Input: part model. Units: mm. Frame: model coordinates. A direction names the side the tool comes from. Round coordinates to 2 decimals unless told otherwise and drop trailing zeros. Order: outer loops, then holes, each group sorted by start corner. A loop starts at its lowest first (then second) coordinate and runs counter-clockwise, first axis right, second up. Notation, with made-up numbers: (-8.75, 84) -> (48.25, 84) arc R13 cw to (48.25, 90) -> close; hole circle Ø10 at (73.5, -5). An arc over 180 degrees is marked (long way). Use a Markdown table: item, result.
Autodesk Inventor part; units mm, degrees
ref_plane "YZ Plane" through (0, 0, 0) normal (1, 0, 0) x (0, 1, 0)
ref_plane "XZ Plane" through (0, 0, 0) normal (0, 1, 0) x (-1, 0, 0)
ref_plane "XY Plane" through (0, 0, 0) normal (0, 0, 1) x (1, 0, 0)
sketch "Эскиз1" plane through (0, 0, 0) normal (0, 0, 1) x (1, 0, 0)
  line L0 (0, 0) -> (-40, 0)
  line L1 (-40, -30) -> (-30, -30)
  line L2 (-30, -30) -> (-30, -34)
  line L3 (-30, -34) -> (-10, -34)
  line L4 (-10, -34) -> (-10, -30)
  line L5 (-10, -30) -> (0, -30)
  line L6 (-40, -30) -> (-40, -15)
  line L7 (-40, -15) -> (-32, -15)
  line L8 (-32, -15) -> (-32, 0)
  line L9 (-40, 30) -> (-30, 30)
  line L10 (-30, 30) -> (-30, 34)
  line L11 (-30, 34) -> (-10, 34)
  line L12 (-10, 34) -> (-10, 30)
  line L13 (-10, 30) -> (0, 30)
  line L14 (-40, 30) -> (-40, 15)
  line L15 (-40, 15) -> (-32, 15)
  line L16 (-32, 15) -> (-32, 0)
  line L17 (0, 30) -> (0, -30)
  line L18 (0, 0) -> (40, 0)
  line L19 (40, -30) -> (30, -30)
  line L20 (30, -30) -> (30, -34)
  line L21 (30, -34) -> (10, -34)
  line L22 (10, -34) -> (10, -30)
  line L23 (10, -30) -> (0, -30)
  line L24 (40, -30) -> (40, -15)
  line L25 (40, -15) -> (32, -15)
  line L26 (32, -15) -> (32, 0)
  line L27 (40, 30) -> (30, 30)
  line L28 (30, 30) -> (30, 34)
  line L29 (30, 34) -> (10, 34)
  line L30 (10, 34) -> (10, 30)
  line L31 (10, 30) -> (0, 30)
  line L32 (40, 30) -> (40, 15)
  line L33 (40, 15) -> (32, 15)
  line L34 (32, 15) -> (32, 0)
  dimension "d0" = 4
  dimension "d1" = 60
  dimension "d3" = 20
  dimension "d6" = 15
  dimension "d8" = 15
  dimension "d9" = 10
  dimension "d11" = 20
  dimension "d14" = 8
extrude "Выдавливание1" add sketch "Эскиз1" along normal blind 4
sketch "Эскиз2" plane through (0, 0, 4) normal (0, 0, 1) x (1, 0, 0)
  line L0 (10, 30) -> (-10, 30)
  line L1 (0, 30) -> (0, -30)
  line L2 (-10, -30) -> (10, -30)
  line L3 (-32, 15) -> (-32, -15)
  line L4 (-32, 0) -> (32, 0)
  line L5 (32, -15) -> (32, 15)
  line L6 (-40, 15) -> (-32, 15)
  line L7 (-30, 30) -> (-40, 30)
  line L8 (-40, 30) -> (-40, 15)
  point P0 (0, 0)
  point P1 (-36, -21)
  point P2 (36, -21)
  point P3 (-36, 21)
  point P4 (36, 21)
  point P5 (-36, 15)
  point P6 (-40, 22.5)
  dimension "d23" = 9
hole "Отверстие1" at (-36, -21, 4) at (36, -21, 4) at (-36, 21, 4) at (36, 21, 4) direction (0, 0, -1) diameter 3 end through all
sketch "Эскиз3" plane through (0, 0, 4) normal (0, 0, 1) x (1, 0, 0)
  line L0 (0, 0) -> (0, 30)
  line L1 (10, 30) -> (-10, 30)
  point P0 (-12.8, 10)
  point P1 (12.8, 10)
  dimension "d31" = 25.6
  dimension "d32" = 10
hole "Отверстие2" at (-12.8, 10, 4) at (12.8, 10, 4) direction (0, 0, -1) diameter 16 end through all
sketch "Эскиз4" plane through (0, 0, 4) normal (0, 0, 1) x (1, 0, 0)
  circle A0 centre (-12.8, 10) radius 8
  line L0 (-10, -30) -> (10, -30)
  line L1 (0, -30) -> (0, 30)
  line L2 (10, 30) -> (-10, 30)
  point P0 (0, 0)
  point P1 (-27.5, 10)
  point P2 (27.5, 10)
  dimension "d40" = 55
hole "Отверстие3" at (-27.5, 10, 4) at (27.5, 10, 4) direction (0, 0, -1) diameter 3 end through all
sketch "Эскиз5" plane through (0, 0, 4) normal (0, 0, 1) x (1, 0, 0)
  line L0 (-26, -3) -> (-3, -3)
  line L1 (-3, -3) -> (-3, -8)
  line L2 (-3, -8) -> (-26, -8)
  line L3 (-26, -8) -> (-26, -3)
  line L4 (3, -3) -> (26, -3)
  line L5 (26, -3) -> (26, -8)
  line L6 (26, -8) -> (3, -8)
  line L7 (3, -8) -> (3, -3)
  line L8 (-10, -30) -> (10, -30)
  line L9 (0, -30) -> (0, 30)
  line L10 (10, 30) -> (-10, 30)
  line L11 (32, -15) -> (32, 15)
  point P0 (0, 0)
  point P1 (3, -5.5)
  point P2 (-3, -5.5)
  dimension "d42" = 23
  dimension "d43" = 22
  dimension "d44" = 5
  dimension "d45" = 6
extrude "Выдавливание2" cut sketch "Эскиз5" against normal through all
properties part number "top" material "Дерево (береза)"
1) Cut plane A-A on y = 21. Return loops of the section in (x, z).
Answer key:
| item | result |
|---|---|
| outline | (-40, 0) -> (-37.5, 0) -> (-37.5, 4) -> (-40, 4) -> close; (-34.5, 0) -> (34.5, 0) -> (34.5, 4) -> (-34.5, 4) -> close; (37.5, 0) -> (40, 0) -> (40, 4) -> (37.5, 4) -> close |
2) Contact query for flat-ended pins moving along their axis: P1, Ø2.5, axis at x = 36, y = 21, coming from the -Z side; P2, Ø2, axis at y = -5, z = 3, coming from the +X side; P3, Ø1.2, axis at y = -6, z = 1, coming from the -X side; P4, Ø2, axis at y = 33, z = 2, coming from the +X side. Output: stop coordinate, or through.
Answer key:
| item | result |
|---|---|
| P1 | passes through |
| P2 | stops at x = 32 |
| P3 | stops at x = -32 |
| P4 | stops at x = 30 |
3) Cut plane B-B on x = 36. Return loops of the section in (y, z), and give its area (3 significant figures).
Answer key:
| item | result |
|---|---|
| outline | (-30, 0) -> (-22.5, 0) -> (-22.5, 4) -> (-30, 4) -> close; (-19.5, 0) -> (-15, 0) -> (-15, 4) -> (-19.5, 4) -> close; (15, 0) -> (19.5, 0) -> (19.5, 4) -> (15, 4) -> close; (22.5, 0) -> (30, 0) -> (30, 4) -> (22.5, 4) -> close |
| area | 96.0 mm^2 |
4) Set-up query: faces 4 (the face through (-10, -32, 2)), 5 (the face through (30, -32, 2)), 6 (the face through (-14, -8, 2)). Return all of +Z, -Z, +X, -X, +Y, -Y with unobstructed straight access to the full face (end or side cutting, diameter ignored); none if empty.
Answer key:
| item | result |
|---|---|
| face 4 | +Z, -Z, -Y |
| face 5 | +Z, -Z, +X, -Y |
| face 6 | +Z, -Z |
5) Draft query along Y for faces 1 (the face through (-20, 34, 2)), 2 (the face through (-29, 10, 2)), 3 (the face through (-30, -32, 2)). Return one class per face: released by +Y, released by -Y, zero draft, split by the parting line, or undercut.
Answer key:
| item | result |
|---|---|
| face 1 | released by +Y |
| face 2 | undercut |
| face 3 | zero draft |
6) Cut plane D-D on x = 27.5. Return loops of the section in (y, z).
Answer key:
| item | result |
|---|---|
| outline | (-34, 0) -> (8.5, 0) -> (8.5, 4) -> (-34, 4) -> close; (11.5, 0) -> (34, 0) -> (34, 4) -> (11.5, 4) -> close |
7) Cut plane C-C on x = -12.8. Return loops of the section in (y, z), and give its area (3 significant figures).
Answer key:
| item | result |
|---|---|
| outline | (-34, 0) -> (-8, 0) -> (-8, 4) -> (-34, 4) -> close; (-3, 0) -> (2, 0) -> (2, 4) -> (-3, 4) -> close; (18, 0) -> (34, 0) -> (34, 4) -> (18, 4) -> close |
| area | 188 mm^2 |
8) Ray query, probe 1 along X at (y, z) = (10, 3.3); probe 2 along X at (y, z) = (21, 1.6); probe 3 along Y at (x, z) = (-36, 0.9). Return the intervals inside material, ascending.
Answer key:
| item | result |
|---|---|
| probe 1 | x = -32 to -29, -26 to -20.8, -4.8 to 4.8, 20.8 to 26, 29 to 32 |
| probe 2 | x = -40 to -37.5, -34.5 to 34.5, 37.5 to 40 |
| probe 3 | y = -30 to -22.5, -19.5 to -15, 15 to 19.5, 22.5 to 30 |
